Geometry: final body of the model. Coordinates: model frame, mm. A direction names the side the tool comes from. Coordinates: 2 decimals unless noted, no trailing zeros. Order: outer loops, then holes, each group sorted by start corner. A loop starts at its lowest first (then second) coordinate and runs counter-clockwise, first axis right, second up. Notation, with made-up numbers: (23, 88) -> (70, 88) arc R27 ccw to (70, 110) -> close; hole circle Ø10 at (71, 83). An arc over 180 degrees is marked (long way). Answer in a Markdown table with one row per item. Add a question column.
1) Section query B-B on z = 35. Return the cut outline in (x, y), then the cut area to 3 significant figures.
2) Pull-direction query (Z, two-part tool) for faces 1 (the face through (-18, 0, 10.5)), 2 (the face through (1, 0, 32)), 3 (the face through (-7.9, 0.79, 36.91)); classes: +Z half, -Z half, draft (parallel to the pull), parting line (faces both ways), or undercut.
3) Contact query for flat-ended pins moving along their axis: P1, Ø9, axis at y = -1, z = 32.5, coming from the +X side; P2, Ø7, axis at x = -21, y = 0, coming from the -Z side; P3, Ø10, axis at y = -4, z = 26, coming from the -X side; P4, Ø7, axis at x = 21, y = 0, coming from the +Z side. Output: stop coordinate, or through.
4) Section query A-A on x = 3. Return the cut outline in (y, z), then the cut area to 3 significant figures.
5) Section query D-D on x = -21. Return the cut outline in (y, z).
6) Section query C-C on z = 11.5. Return the cut outline in (x, y), then the cut area to 3 significant figures.
7) Ray query, line 1 (X direction, y = 0, z = 6); line 2 (Z direction, x = -8.75, y = 0); line 3 (Z direction, x = 5.25, y = 0). Return the intervals inside material, ascending. Write a range as from..to.
8) Set-up query: faces 4 (the face through (-1, -2.4, 34.6)), 5 (the face through (18, 0, 10.5)), 6 (the face through (-10, 0, 19)). Return all of +Z, -Z, +X, -X, +Y, -Y with unobstructed straight access to the full face (end or side cutting, diameter ignored); none if empty.
Autodesk Inventor part; units mm, degrees
ref_plane "YZ Plane" through (0, 0, 0) normal (1, 0, 0) x (0, 1, 0)
ref_plane "XZ Plane" through (0, 0, 0) normal (0, 1, 0) x (-1, 0, 0)
ref_plane "XY Plane" through (0, 0, 0) normal (0, 0, 1) x (1, 0, 0)
sketch "スケッチ1" plane through (0, 0, 0) normal (0, 0, 1) x (1, 0, 0)
  line L0 (-26, 10) -> (26, 10)
  line L1 (26, 10) -> (26, -10)
  line L2 (26, -10) -> (-26, -10)
  line L3 (-26, -10) -> (-26, 10)
  point P0 (0, 0)
  point P1 (0, -10)
  point P2 (-26, 0)
  dimension "d0" = 52
  dimension "d1" = 20
extrude "押し出し1" add sketch "スケッチ1" along normal blind 10.5
sketch "スケッチ2" plane through (0, 0, 10.5) normal (0, 0, 1) x (1, 0, 0)
  line L0 (-26, 10) -> (26, 10)
  line L1 (26, -10) -> (-26, -10)
  line L2 (-15, 10) -> (15, 10)
  line L3 (15, 10) -> (15, -10)
  line L4 (15, -10) -> (-15, -10)
  line L5 (-15, -10) -> (-15, 10)
  point P0 (0, 0)
  point P1 (0, -10)
  dimension "d4" = 30
extrude "押し出し2" add sketch "スケッチ2" along normal blind 29.5
sketch "スケッチ4" plane through (-26, -10, 0) normal (0, -1, 0) x (1, 0, 0)
  line L0 (52, 0) -> (0, 0)
  line L1 (16, 29) -> (36, 29)
  line L2 (36, 29) -> (36, 9)
  line L3 (36, 9) -> (16, 9)
  line L4 (16, 9) -> (16, 29)
  point P0 (26, 0)
  point P1 (26, 9)
  point P2 (26, 0)
  dimension "d8" = 20
  dimension "d9" = 20
  dimension "d10" = 9
extrude "押し出し3" cut sketch "スケッチ4" against normal through all
sketch "スケッチ5" plane through (0, 0, 40) normal (0, 0, 1) x (1, 0, 0)
  line L0 (-15, 10) -> (15, 10)
  line L1 (15, -10) -> (-15, -10)
  line L2 (-1, 10) -> (1, 10)
  line L3 (1, 10) -> (1, -10)
  line L4 (1, -10) -> (-1, -10)
  line L5 (-1, -10) -> (-1, 10)
  point P0 (0, 0)
  point P1 (0, -10)
  dimension "d13" = 2
extrude "押し出し4" cut sketch "スケッチ5" against normal up to surface (11 mm away)
sketch "スケッチ6" plane through (0, 0, 10.5) normal (0, 0, 1) x (1, 0, 0)
  line L0 (-26, -10) -> (-26, 10)
  line L1 (26, 10) -> (26, -10)
  point P0 (0, 0)
  point P1 (-21, 0)
  point P2 (21, 0)
  point P3 (-26, 0)
  dimension "d16" = 5
  dimension "d17" = 5
hole "穴1" at (-21, 0, 10.5) at (21, 0, 10.5) direction (0, 0, -1) diameter 5.5 end through all
sketch "スケッチ7" plane through (15, -10, 10.5) normal (1, 0, 0) x (0, 0, -1)
  line L0 (-29.5, 20) -> (-29.5, 0)
  line L1 (10.5, 12.75) -> (10.5, 7.25)
  point P0 (10.5, 10)
  point P1 (-24.5, 10)
  point P2 (-29.5, 10)
  dimension "d25" = 35
hole "穴2" at (15, 0, 35) direction (-1, 0, 0) diameter 5.5 end up to surface counterbore diameter 9.5 counterbore depth 5.5
sketch "スケッチ8" plane through (-15, -10, 10.5) normal (-1, 0, 0) x (0, 0, 1)
  circle A0 centre (24.5, 10) radius 2.75
  point P0 (-10.5, 10)
hole "穴3" at (-15, 0, 35) direction (1, 0, 0) diameter 4.134 end up to surface
chamfer "面取り1" distance 1 angle 45 4 edges at (-26, 10, 5.25) (26, 10, 5.25) (26, -10, 5.25) (-26, -10, 5.25)
equation "\"d9\" = d8"
properties part number "CLTQAM20" material "MISUMI"
Result:
| question | item | result |
|---|---|---|
| 1 | outline | (-15, -10) -> (-1, -10) -> (-1, -2.07) -> (-15, -2.07) -> close; (-15, 2.07) -> (-1, 2.07) -> (-1, 10) -> (-15, 10) -> close; (1, -10) -> (15, -10) -> (15, -4.75) -> (9.5, -4.75) -> (9.5, -2.75) -> (1, -2.75) -> close; (1, 2.75) -> (9.5, 2.75) -> (9.5, 4.75) -> (15, 4.75) -> (15, 10) -> (1, 10) -> close |
| 1 | area | 403 mm2 |
| 2 | face 1 | +Z half |
| 2 | face 2 | draft |
| 2 | face 3 | undercut |
| 3 | P1 | x = 15 |
| 3 | P2 | z = 0 |
| 3 | P3 | x = -15 |
| 3 | P4 | z = 10.5 |
| 4 | outline | (-10, 0) -> (10, 0) -> (10, 9) -> (-10, 9) -> close; (-10, 29) -> (10, 29) -> (10, 40) -> (-10, 40) -> close; hole circle Ø5.5 at (0, 35) |
| 4 | area | 376 mm2 |
| 5 | outline | (-10, 0) -> (-2.75, 0) -> (-2.75, 10.5) -> (-10, 10.5) -> close; (2.75, 0) -> (10, 0) -> (10, 10.5) -> (2.75, 10.5) -> close |
| 6 | outline | (-15, -10) -> (-10, -10) -> (-10, 10) -> (-15, 10) -> close; (10, -10) -> (15, -10) -> (15, 10) -> (10, 10) -> close |
| 6 | area | 200 mm2 |
| 7 | line 1 | -26..-23.75, -18.25..18.25, 23.75..26 |
| 7 | line 2 | 0..9, 29..32.93, 37.07..40 |
| 7 | line 3 | 0..9, 29..32.25, 37.75..40 |
| 8 | face 4 | +Z, +Y, -Y |
| 8 | face 5 | +Z, +X, +Y, -Y |
| 8 | face 6 | +Y, -Y |
